from build123d import *

# Parameters (mm, degrees)
F0_W        = 254
F0_H        = 50.8
F1_DEPTH    = 38.1
F2_T1_DEPTH = 1365.7843192567
F3_W        = 25.5302116275
F3_H        = 25.5302092992
F4_DEPTH    = 76.2


# Not quite as in the source:
# - a fillet or chamfer that OpenCascade refuses, or shapes differently, is made with other operations: its cross-section is extruded or revolved along the edge and cut away or added


with BuildPart() as f1:
    # F0 (on Front) → F1 (new body)
    with BuildSketch(Plane.XZ):
        with Locations((-22.1173410591, 25.4)):
            Rectangle(F0_W, F0_H)
    extrude(amount=F1_DEPTH)

    # F2: chamfer of 50.8 x 255.5053741775 on 1 edges, made by hand

    # F2_s2 → F2_t1 (cut)
    with BuildSketch(Plane.XZ.offset(-663.8421596283)):
        Polygon((106.3880331184, 50.8), (-149.1173410591, 0), (-149.1173410591, 50.8), align=None)
    extrude(amount=F2_T1_DEPTH, mode=Mode.SUBTRACT)

    # F3 (on face) → F4 (join)
    with BuildSketch(Plane.XZ.offset(38.1)):
        with Locations((86.3100104034, 20.4800155479)):
            Rectangle(F3_W, F3_H)
    extrude(amount=F4_DEPTH)


solid = f1.part
Read the model definition and answer for the solid it produces. Units are mm, in the model's axes. A direction names the side the tool comes from. Coordinates: 2 decimals unless noted, no trailing zeros. Order: outer loops, then holes, each group sorted by start corner. A loop starts at its lowest first (then second) coordinate and runs counter-clockwise, first axis right, second up. Notation, with made-up numbers: (88.5, -25) - (97.5, -25) arc R13 cw to (97.5, -9) - close; hole circle Ø2 at (55, 71.25). An arc over 180 degrees is marked (long way). Use one line per item in the form item = value.
(1) Section C-C, the plane x = 87 is taken. Give the vertices of the cut face in (y, z), then the cut area to 3 significant figures.
Computed values:
outline = (-114.3, 7.71) - (-38.1, 7.71) - (-38.1, 0) - (0, 0) - (0, 46.95) - (-38.1, 46.95) - (-38.1, 33.25) - (-114.3, 33.25) - close
area = 3,730 mm²
(2) Section A-A, the plane z = 16 is taken. Give the vertices of the cut face in (x, y).
Computed values:
outline = (-68.64, -38.1) - (73.54, -38.1) - (73.54, -114.3) - (99.08, -114.3) - (99.08, -38.1) - (104.88, -38.1) - (104.88, 0) - (-68.64, 0) - close
(3) Section D-D, the plane y = -32 is taken. Give the vertices of the cut face in (x, z), then the cut area to 3 significant figures.
Computed values:
outline = (-149.12, 0) - (104.88, 0) - (104.88, 50.5) - close
area = 6,410 mm²
(4) Section B-B, the plane y = -73 is taken. Give the vertices of the cut face in (x, z), then the cut area to 3 significant figures.
Computed values:
outline = (73.54, 7.71) - (99.08, 7.71) - (99.08, 33.25) - (73.54, 33.25) - close
area = 652 mm²
(5) Straight lines are drawn through the part: L1, parallel to Y at x = 13.5, z = 26; L2, parallel to X at y = -100, z = 9; L3, parallel to Z at x = 27, y = -25. For each, find the intervals that lie inside material, in ascending order.
Computed values:
L1 = -38.1 to 0
L2 = 73.54 to 99.08
L3 = 0 to 35.02
(6) Which of the six approach directions +Z, -Z, +X, -X, +Y, -Y give full straight-line access (tool end or side, diameter ignored) to faces 1 (the face through (73.545, -76, 20)), 2 (the face through (86, -76, 7.715)), 3 (the face through (-20.339, -18.783, 25.604)), 4 (the face through (86, -76, 33.245)), 5 (the face through (99.075, -76, 20))?
Computed values:
face_1 = +Z, -Z, -X, -Y
face_2 = -Z, +X, -X, -Y
face_3 = +Z, -X, +Y, -Y
face_4 = +Z, +X, -X, -Y
face_5 = +Z, -Z, +X, -Y
(7) Given pin 1 Ø12 at (x, z) = (41.5, 39.5) entering from -Y; pin 2 Ø2 at (y, z) = (-98, 33) entering from +X; pin 3 Ø13 at (x, y) = (91.5, -73) entering from +Z, each flat-ended and moving along its own axis, determine where each tip first touches the part or whether it passes through.
Computed values:
pin_1 = -38.1
pin_2 = 99.08
pin_3 = 33.25
